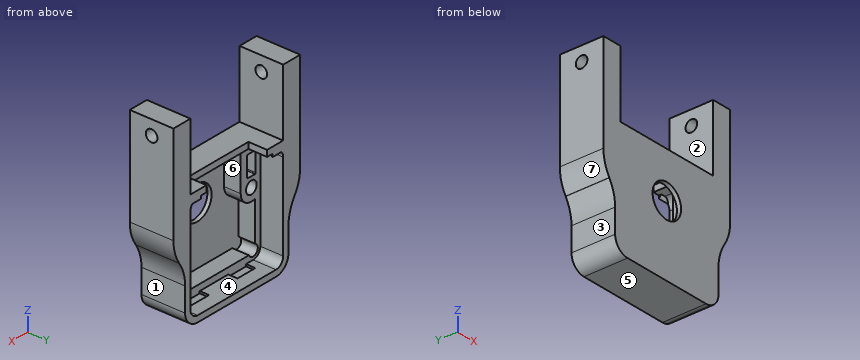
```python
from build123d import *

# Parameters (mm, degrees)
BOSS_EXTRUDE1_DEPTH     = 9.5
BOSS_EXTRUDE2_START     = 1
BOSS_EXTRUDE2_DEPTH     = 1
CUT_EXTRUDE1_DEPTH      = 40.261368341
CUT_EXTRUDE1_DEPTH_BACK = 40.261368341
SKETCH4_R               = 4
SKETCH5_R               = 1.5
BOSS_EXTRUDE3_DEPTH     = 4
CUT_EXTRUDE2_DEPTH      = 41.283880697
CUT_EXTRUDE2_DEPTH_BACK = 3
SKETCH6_W               = 17
SKETCH6_H               = 4.5
BOSS_EXTRUDE4_DEPTH     = 10.5
CUT_EXTRUDE3_DEPTH      = 46.272780922
CUT_EXTRUDE3_DEPTH_BACK = 46.272780922
SKETCH9_R               = 1.4
FILLET1_R               = 10
BOSS_EXTRUDE6_DEPTH     = 3
SKETCH14_W              = 5
SKETCH14_H              = 2.25
CUT_EXTRUDE4_DEPTH      = 0.5


with BuildPart() as part:
    # Sketch1 → Boss-Extrude1 (new body)
    with BuildSketch(Plane(origin=(0, 0, 0), x_dir=(1, 0, 0), z_dir=(0, 1, 0))):
        with BuildLine():
            Line((-1.5, 2), (-1.5, 22.862))
            ThreePointArc((-1.5, 22.862), (-0.474873734, 25.336873734), (2, 26.362))
            Line((2, 26.362), (24, 26.362))
            ThreePointArc((24, 26.362), (26.474873734, 25.336873734), (27.5, 22.862))
            Line((27.5, 22.862), (27.5, 2))
            Line((27.5, 2), (27.5, -1.5))
            Line((27.5, -1.5), (24, -1.5))
            Line((24, -1.5), (2, -1.5))
            Line((2, -1.5), (-1.5, -1.5))
            Line((-1.5, -1.5), (-1.5, 2))
        make_face()
        with BuildLine():
            Line((2, 0), (24, 0))
            ThreePointArc((24, 0), (25.414213562, 0.585786438), (26, 2))
            Line((26, 2), (26, 22.862))
            ThreePointArc((26, 22.862), (25.414213562, 24.276213562), (24, 24.862))
            Line((24, 24.862), (2, 24.862))
            ThreePointArc((2, 24.862), (0.585786438, 24.276213562), (0, 22.862))
            Line((0, 22.862), (0, 2))
            ThreePointArc((0, 2), (0.585786438, 0.585786438), (2, 0))
        make_face(mode=Mode.SUBTRACT)
    extrude(amount=BOSS_EXTRUDE1_DEPTH)

    # Sketch3 → Boss-Extrude2 (add)
    with BuildSketch(Plane.XZ.offset(BOSS_EXTRUDE2_START)):
        with BuildLine():
            Line((24, -26.362), (2, -26.362))
            ThreePointArc((2, -26.362), (-0.474873734, -25.336873734), (-1.5, -22.862))
            Line((-1.5, -22.862), (-1.5, 1.5))
            Line((-1.5, 1.5), (27.5, 1.5))
            Line((27.5, 1.5), (27.5, -22.862))
            ThreePointArc((27.5, -22.862), (26.474873734, -25.336873734), (24, -26.362))
        make_face()
    extrude(amount=-BOSS_EXTRUDE2_DEPTH)

    # Sketch4 → Cut-Extrude1 (cut, two sides: drawn at the far end of the back side and taken through both)
    with BuildSketch(Plane(origin=(0, 0, 0), x_dir=(1, 0, 0), z_dir=(0, 1, 0)).offset(-CUT_EXTRUDE1_DEPTH_BACK)):
        with Locations(Location((13, 9.5, 0), (0, 0, 270))):
            Circle(SKETCH4_R)
    extrude(amount=CUT_EXTRUDE1_DEPTH + CUT_EXTRUDE1_DEPTH_BACK, mode=Mode.SUBTRACT)

    # Sketch5 → Boss-Extrude3 (add)
    with BuildSketch(Plane(origin=(0, 0, 0), x_dir=(1, 0, 0), z_dir=(0, 1, 0))):
        with BuildLine():
            Line((3.2, 23.362), (22.866091564, 23.362))
            ThreePointArc((22.866091564, 23.362), (24.876284298, 23.738284298), (24.5, 21.728091564))
            Line((24.5, 21.728091564), (24.5, 12.199689562))
            ThreePointArc((24.5, 12.199689562), (21.767949192, 11.82075218), (20.5, 9.371262437))
            Line((20.5, 9.371262437), (20.5, 0))
            Line((20.5, 0), (24, 0))
            ThreePointArc((24, 0), (25.414213562, 0.585786438), (26, 2))
            Line((26, 2), (26, 22.862))
            ThreePointArc((26, 22.862), (25.414213562, 24.276213562), (24, 24.862))
            Line((24, 24.862), (2, 24.862))
            ThreePointArc((2, 24.862), (0.585786438, 24.276213562), (0, 22.862))
            Line((0, 22.862), (0, 2))
            ThreePointArc((0, 2), (0.585786438, 0.585786438), (2, 0))
            Line((2, 0), (5.5, 0))
            Line((5.5, 0), (5.5, 9.371262437))
            ThreePointArc((5.5, 9.371262437), (4.232050808, 11.82075218), (1.5, 12.199689562))
            Line((1.5, 12.199689562), (1.5, 21.662))
            ThreePointArc((1.5, 21.662), (1.080761184, 23.781238816), (3.2, 23.362))
        make_face()
        with BuildLine():
            Line((3.5, 2), (1.5, 2))
            ThreePointArc((1.5, 2), (1.358578644, 2.058578644), (1.3, 2.2))
            Line((1.3, 2.2), (1.3, 6.8))
            ThreePointArc((1.3, 6.8), (1.358578644, 6.941421356), (1.5, 7))
            Line((1.5, 7), (3.5, 7))
            ThreePointArc((3.5, 7), (3.641421356, 6.941421356), (3.7, 6.8))
            Line((3.7, 6.8), (3.7, 2.2))
            ThreePointArc((3.7, 2.2), (3.641421356, 2.058578644), (3.5, 2))
        make_face(mode=Mode.SUBTRACT)
        with Locations(Location((2.5, 9.371262437, 0), (0, 0, 270))):
            Circle(SKETCH5_R, mode=Mode.SUBTRACT)
        with BuildLine():
            ThreePointArc((22.5, 2), (22.358578644, 2.058578644), (22.3, 2.2))
            Line((22.3, 2.2), (22.3, 6.8))
            ThreePointArc((22.3, 6.8), (22.358578644, 6.941421356), (22.5, 7))
            Line((22.5, 7), (24.5, 7))
            ThreePointArc((24.5, 7), (24.641421356, 6.941421356), (24.7, 6.8))
            Line((24.7, 6.8), (24.7, 2.2))
            ThreePointArc((24.7, 2.2), (24.641421356, 2.058578644), (24.5, 2))
            Line((24.5, 2), (22.5, 2))
        make_face(mode=Mode.SUBTRACT)
        with Locations(Location((23.5, 9.371262437, 0), (0, 0, 90))):
            Circle(SKETCH5_R, mode=Mode.SUBTRACT)
    extrude(amount=BOSS_EXTRUDE3_DEPTH)

    # Sketch6 → Cut-Extrude2 (cut, two sides: drawn at the far end of the back side and taken through both)
    with BuildSketch(Plane.XY.offset(1.5).offset(-CUT_EXTRUDE2_DEPTH_BACK)):
        with Locations((13, 7.25)):
            Rectangle(SKETCH6_W, SKETCH6_H)
    extrude(amount=CUT_EXTRUDE2_DEPTH + CUT_EXTRUDE2_DEPTH_BACK, mode=Mode.SUBTRACT)

    # Sketch7 → Boss-Extrude4 (add)
    with BuildSketch(Plane.XZ.offset(1)):
        Polygon((27.5, -14.163598373), (30.779339473, -9.127595345), (30.779339473, 17.5), (26, 17.5), (26, 1.5), (27.5, 1.5), align=None)
    boss_extrude4 = extrude(amount=-BOSS_EXTRUDE4_DEPTH)

    # Mirror1: Boss-Extrude4 across plane
    add(boss_extrude4.mirror(Plane(origin=(13, 0, 0), x_dir=(0, 0, 1), z_dir=(1, 0, 0))))

    # Sketch9 → Cut-Extrude3 (cut, two sides: drawn at the far end of the back side and taken through both)
    with BuildSketch(Plane.ZY.offset(4.779339473).offset(-CUT_EXTRUDE3_DEPTH_BACK)):
        with Locations((14, 4.25)):
            Circle(SKETCH9_R)
    extrude(amount=CUT_EXTRUDE3_DEPTH + CUT_EXTRUDE3_DEPTH_BACK, mode=Mode.SUBTRACT)

    # Fillet1
    fillet1_edges = [part.edges().sort_by_distance(p)[0] for p in [
        (30.779339473, 4.25, -9.127595345),
        (27.5, 4.25, -14.163598373),
        (-1.5, 4.25, -14.163598373),
        (-4.779339473, 4.25, -9.127595345),
    ]]
    fillet(fillet1_edges, radius=FILLET1_R)

    # Sketch13 → Boss-Extrude6 (add)
    with BuildSketch(Plane(origin=(0, 0, 0), x_dir=(0, 0, -1), z_dir=(1, 0, 0))):
        Polygon((0, 9.5), (0.7, 9.5), (0, 8.9), align=None)
    boss_extrude6 = extrude(amount=BOSS_EXTRUDE6_DEPTH)

    # Sketch14 → Cut-Extrude4 (cut)
    with BuildSketch(Plane.XY.offset(-24.862)):
        with Locations((6.5, 5.125)):
            Rectangle(SKETCH14_W, SKETCH14_H)
    cut_extrude4 = extrude(amount=-CUT_EXTRUDE4_DEPTH, mode=Mode.SUBTRACT)

    # Mirror3: Boss-Extrude6, Cut-Extrude4 across plane
    add(boss_extrude6.mirror(Plane(origin=(13, 0, 0), x_dir=(0, 0, 1), z_dir=(1, 0, 0))))
    add(cut_extrude4.mirror(Plane(origin=(13, 0, 0), x_dir=(0, 0, 1), z_dir=(1, 0, 0))), mode=Mode.SUBTRACT)


solid = part.part
```
Here's how the part is built. I have some questions about the finished solid (model axes, mm). Face numbers are marked on the shaded views. A direction names the side the tool comes from. Round coordinates to 2 decimals unless told otherwise and drop trailing zeros. Loops run counter-clockwise (first coordinate to the right, second up) from the corner with the lowest first, then second, coordinate; pieces in that order, holes last. Notation, with made-up numbers: (48, -20.5) -> (79, -20.5) arc R18 ccw to (79, -6.5) -> close; hole circle Ø2 at (21.5, -17). An arc over 180 degrees is marked (long way). Answer as CSV lines item,"result". Start each with the question number.
1. For the marked faces 1, 2, 3 and 4, which set-ups out of +Z, -Z, +X, -X, +Y, -Y let a thin tool reach every point of the face, with its end or its side?
2. Imagine slicing it at B-B on x = 13. Write out the boundary of the cut face in (y, z), plus the area to 3 significant figures.
3. I need wall thicknesses on probe 1 along X at (y, z) = (0.25, -4.5); probe 2 along Z at (x, y) = (12, 1.5); probe 3 along Z at (x, y) = (3.5, 0.75). Which ranges of each line are inside material? Lowest first, please. Write a range as from..to.
4. If we mould it in two halves opening along X, with no side actions, what happens to the marked faces 5, 6 and 7? For each: pulls with the +X half, pulls with the -X half, needs draft (parallel to the pull), parting line crosses it, or undercut.
5. Imagine slicing it at D-D on x = 19. Write out the boundary of the cut face in (y, z).
6. Imagine slicing it at A-A on z = 14. Write out the boundary of the cut face in (x, y).
7. I'm going to push flat-ended pins straight in: P1, Ø1.1, axis at x = 20.5, y = 5, coming from the +Z side; P2, Ø2.5, axis at x = 23.5, z = -4, coming from the +Y side; P3, Ø6, axis at y = 6, z = -16.5, coming from the -X side. Where does each tip first touch, or does it pass through?
8. Imagine slicing it at C-C on y = 2.25. State how many separate pieces and enclosed holes the cut face has, plus the area to 3 significant figures.
Solution:
1,face 1,"-Z, +X, +Y, -Y"
1,face 2,"+Z, +Y, -Y"
1,face 3,"-Z, -X, +Y, -Y"
1,face 4,"+Y"
2,outline,"(-1, -26.36) -> (9.5, -26.36) -> (9.5, -24.86) -> (4, -24.86) -> (4, -23.36) -> (0, -23.36) -> (0, -13.5) -> (-1, -13.5) -> close; (-1, -5.5) -> (0, -5.5) -> (0, 0) -> (5, 0) -> (5, 1.5) -> (-1, 1.5) -> close"
2,area,"47.6 mm²"
3,probe 1,"-4.78..1.3, 3.7..5.5, 20.5..22.3, 24.7..30.78"
3,probe 2,"-26.36..-23.36, 0..1.5"
3,probe 3,"-26.36..-23.36, -12.2..-10.49, -8.25..-7, -2..1.5"
4,face 5,"needs draft"
4,face 6,"undercut"
4,face 7,"pulls with the -X half"
5,outline,"(-1, -26.36) -> (9.5, -26.36) -> (9.5, -24.86) -> (6.25, -24.86) -> (6.25, -25.36) -> (4, -25.36) -> (4, -23.36) -> (0, -23.36) -> (0, 0) -> (5, 0) -> (5, 1.5) -> (-1, 1.5) -> close"
6,outline,"(-4.78, -1) -> (0, -1) -> (0, 2.85) -> (-4.78, 2.85) -> close; (-4.78, 5.65) -> (0, 5.65) -> (0, 9.5) -> (-4.78, 9.5) -> close; (26, -1) -> (30.78, -1) -> (30.78, 2.85) -> (26, 2.85) -> close; (26, 5.65) -> (30.78, 5.65) -> (30.78, 9.5) -> (26, 9.5) -> close"
7,P1,"z = 1.5"
7,P2,"y = 4"
7,P3,"x = -2.18"
8,separate pieces,"1"
8,enclosed holes,"5"
8,area,"557 mm²"
